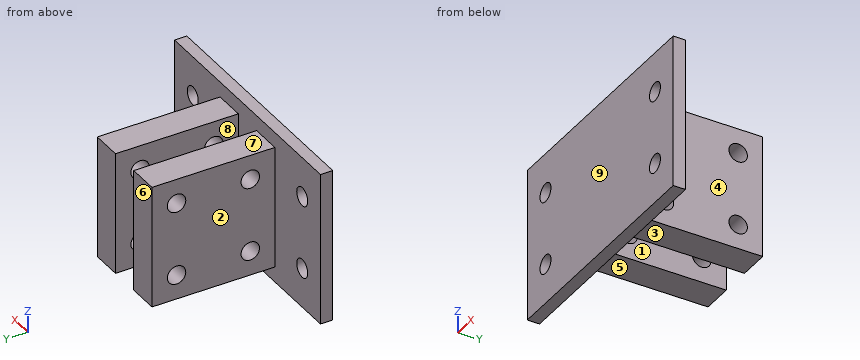
```python
from build123d import *

# Parameters (mm, degrees)
SKETCH_1_W          = 40
SKETCH_1_H          = 25
EXTRUDE_2_DEPTH     = 2
SKETCH_3_W          = 15
SKETCH_3_H          = 20
EXTRUDE_3_DEPTH     = 20
SKETCH_4_W          = 5
SKETCH_4_H          = 20
CUT_EXTRUDE_1_DEPTH = 20
SKETCH_5_R          = 1.5
CUT_EXTRUDE_2_DEPTH = 15
SKETCH_6_R          = 1.5
CUT_EXTRUDE_3_DEPTH = 15


with BuildPart() as part:
    # 草图1 → 凸台-拉伸2 (new body)
    with BuildSketch(Plane(origin=(0, 0, 0), x_dir=(1, 0, 0), z_dir=(0, 1, 0))):
        Rectangle(SKETCH_1_W, SKETCH_1_H)
    extrude(amount=EXTRUDE_2_DEPTH)

    # 草图3 → 凸台-拉伸3 (add)
    with BuildSketch(Plane(origin=(0, 2, 0), x_dir=(1, 0, 0), z_dir=(0, 1, 0))):
        Rectangle(SKETCH_3_W, SKETCH_3_H)
    extrude(amount=EXTRUDE_3_DEPTH)

    # 草图4 → 切除-拉伸1 (cut)
    with BuildSketch(Plane(origin=(0, 22, 0), x_dir=(1, 0, 0), z_dir=(0, 1, 0))):
        Rectangle(SKETCH_4_W, SKETCH_4_H)
    extrude(amount=-CUT_EXTRUDE_1_DEPTH, mode=Mode.SUBTRACT)

    # 草图5 → 切除-拉伸2 (cut)
    with BuildSketch(Plane(origin=(7.5, 0, 0), x_dir=(0, 0, -1), z_dir=(1, 0, 0))):
        with Locations((-6, 18)):
            Circle(SKETCH_5_R)
        with Locations((6, 18)):
            Circle(SKETCH_5_R)
        with Locations((-6, 6)):
            Circle(SKETCH_5_R)
        with Locations((6, 6)):
            Circle(SKETCH_5_R)
    extrude(amount=-CUT_EXTRUDE_2_DEPTH, mode=Mode.SUBTRACT)

    # 草图6 → 切除-拉伸3 (cut)
    with BuildSketch(Plane(origin=(0, 2, 0), x_dir=(1, 0, 0), z_dir=(0, 1, 0))):
        with Locations(Location((-15, 6, 0), (0, 0, 270))):
            Circle(SKETCH_6_R)
        with Locations(Location((-15, -6, 0), (0, 0, 270))):
            Circle(SKETCH_6_R)
        with Locations(Location((15, 6, 0), (0, 0, 270))):
            Circle(SKETCH_6_R)
        with Locations(Location((15, -6, 0), (0, 0, 270))):
            Circle(SKETCH_6_R)
    extrude(amount=-CUT_EXTRUDE_3_DEPTH, mode=Mode.SUBTRACT)


solid = part.part
```
CAD build for the part. Positions are in the model's coordinates, mm. Face numbers are marked on the shaded views. A direction names the side the tool comes from. Round coordinates to 2 decimals unless told otherwise and drop trailing zeros. Write each loop counter-clockwise with the first axis right and the second up, starting at its lowest first coordinate (ties: lowest second). Pieces come first, ordered by that corner, then holes. Notation, with made-up numbers: (76, -21.5) -> (95, -21.5) arc R16 cw to (95, -8.5) -> close; hole circle Ø2 at (9, -32.5). An arc over 180 degrees is marked (long way). Answer in a Markdown table with one row per item. Add a question column.
Item 1: Drill centre lines: line 1 (Y direction, x = 5.4, z = -6); line 2 (X direction, y = 0.7, z = -6); line 3 (Z direction, x = -3, y = 17). Where is each one in solid material? Low to high. Write a range as from..to.
Item 2: Drop flat-ended pins along their axis: pin 1 Ø6 at (x, y) = (14, 7.5) entering from -Z (3 decimals); pin 2 Ø3 at (y, z) = (12.5, 1.5) entering from -X; pin 3 Ø1 at (x, z) = (12, -6.5) entering from +Y; pin 4 Ø2 at (x, y) = (-4, 13.5) entering from +Z. Give the stop position or say it passes through.
Item 3: Saw through at D-D, the plane x = 7. Write the cut outline in (y, z).
Item 4: Saw through at B-B, the plane x = -15. Write the cut outline in (y, z), then the cut area to 3 significant figures.
Item 5: Which spindle directions (+Z, -Z, +X, -X, +Y, -Y) get a long thin tool onto all of the face, cutting with end or side? Do the marked faces 5, 6, 7, 8 and 9. Say none if no direction does.
Item 6: Saw through at A-A, the plane y = 6. Write the cut outline in (x, z), then the cut area to 3 significant figures.
Item 7: Saw through at C-C, the plane z = -6. Count the separate pieces of the cut face and the enclosed holes in it, then the cut area to 3 significant figures.
Item 8: Mould opens along X. For the marked faces 1, 2, 3 and 4 say: pulls with the +X half, pulls with the -X half, needs draft (parallel to the pull), parting line crosses it, or undercut.
Findings below:
| question | item | result |
|---|---|---|
| 1 | line 1 | y = 0..4.5, 7.5..16.5, 19.5..22 |
| 1 | line 2 | x = -20..-16.5, -13.5..13.5, 16.5..20 |
| 1 | line 3 | z = -10..-7.12, -4.88..4.88, 7.12..10 |
| 2 | pin 1 | passes through |
| 2 | pin 2 | stops at x = -7.5 |
| 2 | pin 3 | stops at y = 2 |
| 2 | pin 4 | stops at z = 10 |
| 3 | outline | (0, -12.5) -> (2, -12.5) -> (2, -10) -> (22, -10) -> (22, 10) -> (2, 10) -> (2, 12.5) -> (0, 12.5) -> close; hole circle Ø3 at (6, -6); hole circle Ø3 at (6, 6); hole circle Ø3 at (18, -6); hole circle Ø3 at (18, 6) |
| 4 | outline | (0, -12.5) -> (2, -12.5) -> (2, -7.5) -> (0, -7.5) -> close; (0, -4.5) -> (2, -4.5) -> (2, 4.5) -> (0, 4.5) -> close; (0, 7.5) -> (2, 7.5) -> (2, 12.5) -> (0, 12.5) -> close |
| 4 | area | 38.0 mm^2 |
| 5 | face 5 | -Z, +X, -X, +Y |
| 5 | face 6 | +Z, -Z, +X, -X, +Y |
| 5 | face 7 | +Z, +X, -X, +Y |
| 5 | face 8 | +Z, -Z, +Y |
| 5 | face 9 | +Z, -Z, +X, -X, -Y |
| 6 | outline | (-7.5, -10) -> (-2.5, -10) -> (-2.5, -7.5) -> (-7.5, -7.5) -> close; (-7.5, -4.5) -> (-2.5, -4.5) -> (-2.5, 4.5) -> (-7.5, 4.5) -> close; (-7.5, 7.5) -> (-2.5, 7.5) -> (-2.5, 10) -> (-7.5, 10) -> close; (2.5, -10) -> (7.5, -10) -> (7.5, -7.5) -> (2.5, -7.5) -> close; (2.5, -4.5) -> (7.5, -4.5) -> (7.5, 4.5) -> (2.5, 4.5) -> close; (2.5, 7.5) -> (7.5, 7.5) -> (7.5, 10) -> (2.5, 10) -> close |
| 6 | area | 140 mm^2 |
| 7 | separate pieces | 7 |
| 7 | enclosed holes | 0 |
| 7 | area | 208 mm^2 |
| 8 | face 1 | undercut |
| 8 | face 2 | pulls with the -X half |
| 8 | face 3 | needs draft |
| 8 | face 4 | pulls with the +X half |
